Build history of the part. All positions in model axes, mm. Face numbers are marked on the shaded views. A direction names the side the tool comes from. Give positions to 0.01 mm unless a question says otherwise; leave off trailing zeros. Order: outer loops, then holes, each group sorted by start corner. A loop starts at its lowest first (then second) coordinate and runs counter-clockwise, first axis right, second up. Notation, with made-up numbers: (-2.75, 18) -> (43.25, 18) arc R16 ccw to (43.25, 25) -> close; hole circle Ø9 at (-35, 35). An arc over 180 degrees is marked (long way). One line per item, written item: value. Start each with the question number.
(1) Pin check, flat tips, straight feed: pin 1 (6.5 mm diameter, centred on x = 21.5, y = -16, fed in from -Z); pin 2 (1.5 mm diameter, centred on x = 6, z = 25.5, fed in from -Y); pin 3 (1.5 mm diameter, centred on y = -16, z = 28.5, fed in from +X); pin 4 (3 mm diameter, centred on x = 22.875, y = -13.5, fed in from -Z). Stop position of each tip, or through.
(2) Two-plate mould, pull along X, no slides. Class the marked faces 6, 7 and 8: +X half, -X half, draft (parallel to the pull), parting line (faces both ways), or undercut.
(3) Saw through at C-C on z = 15. Give the cut face in (x, y).
(4) Saw through at B-B on x = 14. Give the cut face in (y, z).
(5) Which spindle directions (+Z, -Z, +X, -X, +Y, -Y) get a long thin tool onto all of the face, cutting with end or side? Do the marked faces 1, 2, 3, 4 and 5. Say none if no direction does.
(6) Probe line 1 (Y direction, x = 12, z = 8.75); line 2 (Z direction, x = 18, y = -11.25); line 3 (Y direction, x = 24, z = 28.5). List the from-to ranges inside material, lowest first.
(7) Saw through at D-D on x = 23. Give the cut face in (y, z).
(8) Saw through at A-A on y = -13.5. Give the cut face in (x, z) (3 decimals).
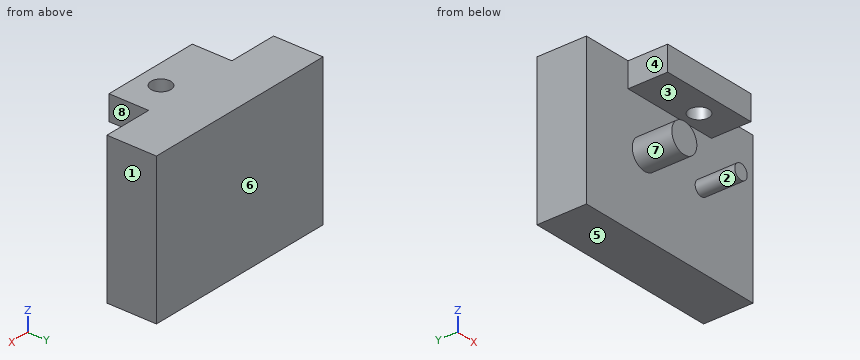
```python
from build123d import *

# Parameters (mm, degrees)
F0_W     = 40
F0_H     = 30
F1_DEPTH = 10
F2_R     = 3
F2_R_2   = 1.5
F2_W     = 20
F2_H     = 5
F3_DEPTH = 8
F4_R     = 2
F5_DEPTH = 5


with BuildPart() as f1:
    # F0 (on Front) → F1 (new body)
    with BuildSketch(Plane.XZ):
        with Locations((20, 15)):
            Rectangle(F0_W, F0_H)
    extrude(amount=F1_DEPTH)

    # F2 (on face) → F3 (join)
    with BuildSketch(Plane.XZ.offset(10)):
        with Locations((14, 15)):
            Circle(F2_R)
        with Locations((27.6, 15)):
            Circle(F2_R_2)
        with Locations((20, 27.5)):
            Rectangle(F2_W, F2_H)
    extrude(amount=F3_DEPTH)

    # F4 (on face) → F5 (cut, through all)
    with BuildSketch(Plane.XY.offset(30)):
        with Locations((22.875, -13.5)):
            Circle(F4_R)
    extrude(amount=-F5_DEPTH, mode=Mode.SUBTRACT)


solid = f1.part
```
Results below:
1. pin 1: stops at z = 25
1. pin 2: stops at y = -10
1. pin 3: stops at x = 30
1. pin 4: passes through
2. face 6: draft
2. face 7: undercut
2. face 8: +X half
3. outline: (0, -10) -> (11, -10) -> (11, -18) -> (17, -18) -> (17, -10) -> (26.1, -10) -> (26.1, -18) -> (29.1, -18) -> (29.1, -10) -> (40, -10) -> (40, 0) -> (0, 0) -> close
4. outline: (-18, 12) -> (-10, 12) -> (-10, 0) -> (0, 0) -> (0, 30) -> (-18, 30) -> (-18, 25) -> (-10, 25) -> (-10, 18) -> (-18, 18) -> close
5. face 1: +Z, -Z, +X, +Y, -Y
5. face 2: -Y
5. face 3: +X, -X, -Y
5. face 4: +Z, -Z, -X, -Y
5. face 5: -Z, +X, -X, +Y, -Y
6. line 1: y = -10 to 0
6. line 2: z = 25 to 30
6. line 3: y = -18 to -15.15, -11.85 to 0
7. outline: (-18, 25) -> (-15.5, 25) -> (-15.5, 30) -> (-18, 30) -> close; (-11.5, 25) -> (-10, 25) -> (-10, 0) -> (0, 0) -> (0, 30) -> (-11.5, 30) -> close
8. outline: (10, 25) -> (20.875, 25) -> (20.875, 30) -> (10, 30) -> close; circle Ø6 at (14, 15); (24.875, 25) -> (30, 25) -> (30, 30) -> (24.875, 30) -> close; circle Ø3 at (27.6, 15)
